Model file for the job. Use its own axes, mm. A direction names the side the tool comes from. Round coordinates to 2 decimals unless told otherwise and drop trailing zeros. Order: outer loops, then holes, each group sorted by start corner. A loop starts at its lowest first (then second) coordinate and runs counter-clockwise, first axis right, second up. Notation, with made-up numbers: M -14,16.5 L 16,16.5 A15 ccw 16,37.5 Z; hole C 21.25,32.25 d5. An arc over 180 degrees is marked long. Return JSON: item names as keys, results as strings. Group by question number.
Item 1: Slice it at A-A on z = 0. Write the cut outline in (x, y) (1 decimal).
Item 2: Slice it at B-B on x = 25.4. Write the cut outline in (y, z) (3 decimals), then the cut area to 3 significant figures.
Item 3: Probe line 1 along X through (y, z) = (2.4, 0) (1 decimal); line 2 along X through (y, z) = (0.6, -12). List the from-to ranges inside material, lowest first.
Item 4: Pull direction Z, two halves, no side cores. Call faces 1 (the face through (-1, 3.175, -1)), 2 (the face through (-1, 2, 38.1)), 3 (the face through (1.588, 2, 0)): pulls with the +Z half, pulls with the -Z half, needs draft (parallel to the pull), parting line crosses it, or undercut.
Item 5: Slice it at C-C on y = 2.45. Give the number of separate pieces and of enclosed holes in the cut face, then the cut area to 3 significant figures.
Item 6: Which spindle directions (+Z, -Z, +X, -X, +Y, -Y) get a long thin tool onto all of the face, cutting with end or side? Do faces 4 (the face through (-50.8, 2, 1)), 5 (the face through (3, 2, 12.7)). Say none if no direction does.
from build123d import *

# Parameters (mm, degrees)
SKETCH2_W           = 101.6
SKETCH2_H           = 76.2
SKETCH2_R           = 3.175
SKETCH2_W_2         = 3.175
SKETCH2_H_2         = 25.4
BOSS_EXTRUDE1_DEPTH = 3.175


with BuildPart() as part:
    # Sketch2 → Boss-Extrude1 (new body)
    with BuildSketch(Plane(origin=(0, 0, 0), x_dir=(1, 0, 0), z_dir=(0, 1, 0))):
        Rectangle(SKETCH2_W, SKETCH2_H)
        with Locations(Location((25.4, 0, 0), (0, 0, 270))):
            Circle(SKETCH2_R, mode=Mode.SUBTRACT)
        with Locations(Location((-25.4, 0, 0), (0, 0, 270))):
            Circle(SKETCH2_R, mode=Mode.SUBTRACT)
        with Locations((3.175, 0)):
            Rectangle(SKETCH2_W_2, SKETCH2_H_2, mode=Mode.SUBTRACT)
        with Locations((-3.175, 0)):
            Rectangle(SKETCH2_W_2, SKETCH2_H_2, mode=Mode.SUBTRACT)
    extrude(amount=BOSS_EXTRUDE1_DEPTH)


solid = part.part
Output values:
{
 "1": {"outline": "M -50.8,0 L -28.6,0 L -28.6,3.2 L -50.8,3.2 Z; M -22.2,0 L -4.8,0 L -4.8,3.2 L -22.2,3.2 Z; M -1.6,0 L 1.6,0 L 1.6,3.2 L -1.6,3.2 Z; M 4.8,0 L 22.2,0 L 22.2,3.2 L 4.8,3.2 Z; M 28.6,0 L 50.8,0 L 50.8,3.2 L 28.6,3.2 Z"},
 "2": {"outline": "M 0,-38.1 L 3.175,-38.1 L 3.175,-3.175 L 0,-3.175 Z; M 0,3.175 L 3.175,3.175 L 3.175,38.1 L 0,38.1 Z", "area": "222 mm²"},
 "3": {"line 1": "-50.8 to -28.6, -22.2 to -4.8, -1.6 to 1.6, 4.8 to 22.2, 28.6 to 50.8", "line 2": "-50.8 to -4.76, -1.59 to 1.59, 4.76 to 50.8"},
 "4": {"face 1": "needs draft", "face 2": "pulls with the +Z half", "face 3": "undercut"},
 "5": {"separate pieces": "1", "enclosed holes": "4", "area": "7,520 mm²"},
 "6": {"face 4": "+Z, -Z, -X, +Y, -Y", "face 5": "+Y, -Y"}
}
